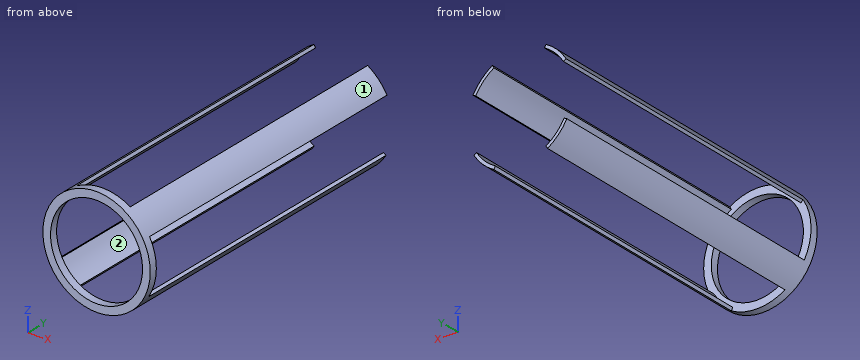
from build123d import *

# Parameters (mm, degrees)
SKETCH2_R               = 88.9
SKETCH2_R_2             = 83.82
BOSS_EXTRUDE1_DEPTH     = 254
CUT_EXTRUDE1_DEPTH      = 255
CUT_EXTRUDE1_DEPTH_BACK = 255
SKETCH4_R               = 88.9
SKETCH4_R_2             = 76.2
BOSS_EXTRUDE2_DEPTH     = 12.7


with BuildPart() as part:
    # Sketch2 → Boss-Extrude1 (new body, symmetric)
    with BuildSketch(Plane(origin=(0, 0, 0), x_dir=(1, 0, 0), z_dir=(0, 1, 0))):
        Circle(SKETCH2_R)
        Circle(SKETCH2_R_2, mode=Mode.SUBTRACT)
    extrude(amount=BOSS_EXTRUDE1_DEPTH, both=True)

    # Sketch3 → Cut-Extrude1 (cut, two sides)
    with BuildSketch(Plane(origin=(0, 0, 0), x_dir=(1, 0, 0), z_dir=(0, 1, 0))) as cut_extrude1_sk:
        Polygon((169.661755759, -94.300371224), (0, 0), (169.661755759, 101.677593364), align=None)
        Polygon((0, 0), (53.900027233, 96.974944394), (-58.116685864, 96.974944394), align=None)
        Polygon((-123.741299607, 68.777140945), (-123.741299607, -74.157652604), (0, 0), align=None)
        Polygon((-65.840936026, -118.45858783), (0, 0), (70.991745134, -118.45858783), align=None)
    extrude(amount=CUT_EXTRUDE1_DEPTH, mode=Mode.SUBTRACT)
    extrude(cut_extrude1_sk.sketch, amount=-CUT_EXTRUDE1_DEPTH_BACK, mode=Mode.SUBTRACT)

    # Sketch4 → Boss-Extrude2 (add)
    with BuildSketch(Plane.XZ.offset(254)):
        Circle(SKETCH4_R)
        Circle(SKETCH4_R_2, mode=Mode.SUBTRACT)
    extrude(amount=-BOSS_EXTRUDE2_DEPTH)


solid = part.part
Part model, mm, in its own coordinate system. Face numbers are marked on the shaded views. Give positions to 0.01 mm unless a question says otherwise; leave off trailing zeros. Order: outer loops, then holes, each group sorted by start corner. A loop starts at its lowest first (then second) coordinate and runs counter-clockwise, first axis right, second up. Notation, with made-up numbers: (-17, -21.75) - (11, -21.75) arc R9 cw to (11, -4.75) - close; hole circle Ø3 at (-1, 80.25). An arc over 180 degrees is marked (long way). Use a Markdown table: item, result.
1) Flat gauge pins, fed straight in: P1, Ø1.5, axis at y = 50, z = 39, coming from the -X side; P2, Ø2, axis at y = -92, z = -67, coming from the +X side; P3, Ø5, axis at y = 81, z = 64.5, coming from the -X side; P4, Ø10, axis at y = -175, z = -59, coming from the +X side. Where does each tip first touch, or does it go through?
Checked values:
| item | result |
|---|---|
| P1 | through |
| P2 | x = 59.56 |
| P3 | x = -63.71 |
| P4 | x = 70.62 |
2) Saw through at D-D on z = -65.5. List the corners of the cut face in (x, y), plus the area to 3 significant figures.
Checked values:
| item | result |
|---|---|
| outline | (-60.11, -254) - (-38.94, -254) - (-38.94, -241.3) - (-52.3, -241.3) - (-52.3, 254) - (-60.11, 254) - close; (38.94, -254) - (60.11, -254) - (60.11, 254) - (52.3, 254) - (52.3, -241.3) - (38.94, -241.3) - close |
| area | 8,270 mm² |
3) Saw through at C-C on z = 0. List the corners of the cut face in (x, y).
Checked values:
| item | result |
|---|---|
| outline | (-88.9, -254) - (-76.2, -254) - (-76.2, -241.3) - (-88.9, -241.3) - close; (76.2, -254) - (88.9, -254) - (88.9, -241.3) - (76.2, -241.3) - close |
4) Saw through at A-A on y = 130.5. List the corners of the cut face in (x, z), plus the area to 3 significant figures.
Checked values:
| item | result |
|---|---|
| outline | (-77.7, -43.19) arc R88.9 ccw to (-45.7, -76.25) - (-43.09, -71.9) arc R83.82 cw to (-73.26, -40.72) - close; (-76.25, 45.7) - (-71.9, 43.09) arc R83.82 cw to (-40.72, 73.26) - (-43.19, 77.7) arc R88.9 ccw to start; (40.72, -73.26) - (43.19, -77.7) arc R88.9 ccw to (76.25, -45.7) - (71.9, -43.09) arc R83.82 cw to start; (43.09, 71.9) arc R83.82 cw to (73.26, 40.72) - (77.7, 43.19) arc R88.9 ccw to (45.7, 76.25) - close |
| area | 919 mm² |
5) Two-plate mould, pull along X, no slides. Class the marked faces 1 and 2: +X half, -X half, draft (parallel to the pull), parting line (faces both ways), or undercut.
Checked values:
| item | result |
|---|---|
| face 1 | parting line |
| face 2 | undercut |
6) Probe L1, parallel to Z at x = 0, y = -248; L2, parallel to Y at x = -79, z = -37.5; L3, parallel to X at y = 103.5, z = -54. List the from-to ranges inside material, lowest first. Write a range as from..to.
Checked values:
| item | result |
|---|---|
| L1 | -88.9..-76.2, 76.2..88.9 |
| L2 | -254..-241.3 |
| L3 | -70.62..-64.11, 64.11..70.62 |
7) Saw through at B-B on x = 0. List the corners of the cut face in (y, z).
Checked values:
| item | result |
|---|---|
| outline | (-254, -88.9) - (-241.3, -88.9) - (-241.3, -76.2) - (-254, -76.2) - close; (-254, 76.2) - (-241.3, 76.2) - (-241.3, 88.9) - (-254, 88.9) - close |
